Autodesk Inventor part; units mm, degrees
ref_plane "YZ Plane" through (0, 0, 0) normal (1, 0, 0) x (0, 1, 0)
ref_plane "XZ Plane" through (0, 0, 0) normal (0, 1, 0) x (-1, 0, 0)
ref_plane "XY Plane" through (0, 0, 0) normal (0, 0, 1) x (1, 0, 0)
sketch "Skizze1" plane through (0, 0, 0) normal (0, 1, 0) x (-1, 0, 0)
  line L0 (10, -8.25) -> (-10, -8.25)
  line L1 (-10, -8.25) -> (-10, 8.25)
  line L2 (-10, 8.25) -> (10, 8.25)
  line L3 (10, 8.25) -> (10, -8.25)
  line L4 (14, 0) -> (-14, 0)
  line L5 (0, -16.2) -> (0, 37.7)
  circle A0 centre (0, -3.25) radius 3
  line L6 (5, 8.25) -> (-5, 8.25)
  line L7 (-5, 8.25) -> (-5, 16.25)
  line L8 (-5, 16.25) -> (5, 16.25)
  line L9 (5, 16.25) -> (5, 8.25)
  point P0 (0, 0)
  point P1 (-5, 8.25)
  dimension "d0" = 20
  dimension "d1" = 16.5
  dimension "d2" = 6
  dimension "d3" = 11.5
  dimension "d13" = 10
  dimension "d14" = 8
extrude "Extrusion1" add sketch "Skizze1" along normal blind 5 contours L0 L5 A0 L4 L3 | L0 L1 L4 L5 A0 | L4 L5 L2 L3 | L4 L1 L2 L5 | L2 L5 L8 L9 | L2 L7 L8 L5
sketch "Skizze2" plane through (0, 5, 0) normal (0, 1, 0) x (1, 0, 0)
  line L0 (10, -8.25) -> (10, 8.25)
  line L1 (10, 8.25) -> (-10, 8.25)
  line L2 (-10, 8.25) -> (-10, -8.25)
  line L3 (-10, -8.25) -> (-5, -8.25)
  circle A0 centre (0, 3.25) radius 3
  line L4 (-2, -8.25) -> (3, -8.25)
  line L5 (-14, 0) -> (14, 0)
  line L6 (0, 16.2) -> (0, -37.7)
  line L7 (-2.5, -18.25) -> (2.5, -18.25)
  line L8 (2.5, -18.25) -> (2.5, -13.25)
  line L9 (2.5, -13.25) -> (-2.5, -13.25)
  line L10 (-2.5, -13.25) -> (-2.5, -18.25)
  line L11 (-5, -8.25) -> (-5, -16.25)
  line L12 (-5, -16.25) -> (5, -16.25)
  line L13 (5, -16.25) -> (5, -8.25)
  line L14 (5, -8.25) -> (10, -8.25)
  circle A1 centre (0, 3.25) radius 3
  circle A2 centre (0, -21.75) radius 4
  circle A3 centre (0, -21.75) radius 8
  line L15 (0, -13.75) -> (0, 3.25)
  point P0 (0, 0)
  dimension "d10" = 5
  dimension "d11" = 5
  dimension "d12" = 5
  dimension "d21" = 8
  dimension "d22" = 25
  dimension "d23" = 4
extrude "Extrusion2" add sketch "Skizze2" against normal blind 60 contours A3 L6 A2 L7 L8 L12 L13 | L13 L12 L8 A3 | L8 L12 L6 A3 | L8 L7 A2 L6 L12 | A3 L11 L12 L10 L7 A2 L6 | L6 L12 L10 A3 | L6 A2 L7 L10 L12 | A3 L10 L12 L11
properties part number "Absicherung Kugellager"
The model under review builds one solid part; all positions refer to its coordinate system, in mm. A direction names the side the tool comes from. Round coordinates to 2 decimals unless told otherwise and drop trailing zeros. Order: outer loops, then holes, each group sorted by start corner. A loop starts at its lowest first (then second) coordinate and runs counter-clockwise, first axis right, second up. Notation, with made-up numbers: (-37.75, 70) - (-18.75, 70) arc R23 ccw to (-18.75, 83) - close; hole circle Ø3 at (81, 77). An arc over 180 degrees is marked (long way). Use one line per item in the form item = value.
Q1. Clearance check with flat-ended pins moving along their axes: P1, Ø10, axis at x = 6, y = -15.5, coming from the -Z side; P2, Ø4, axis at x = -8.5, y = 2, coming from the +Z side; P3, Ø4, axis at x = 6.5, y = 1.5, coming from the +Z side. State where each tip first meets the part, or that it passes through.
Response values:
P1 = 13.81
P2 = 26.41
P3 = 28.36
Q2. Tool access review of faces 1 (the flat face through (-7, 2, 8.25)), 2 (the cylindrical face through (-1.73, -24.58, 29.56)), 3 (the flat face through (5, 2, 12)): name each direction out of +Z, -Z, +X, -X, +Y, -Y from which nothing blocks a thin tool from reaching the whole face with its end or side.
Response values:
face_1 = -X, +Y, -Y
face_2 = -Y
face_3 = +X, +Y, -Y
Q3. To check wall thickness, follow line 1 (Z direction, x = 0, y = 3.45); line 2 (X direction, y = -35.5, z = 21.75); line 3 (X direction, y = 3.85, z = -3.25). State the ranges of each line that lie inside material, in increasing order.
Response values:
line_1 = -8.25 to -6.25, -0.25 to 17.75, 25.75 to 29.75
line_2 = -8 to -4, 4 to 8
line_3 = -10 to -3, 3 to 10
Q4. Add section A-A on z = 21.75. Give the boundary of the cut face in (x, y), then the cut area to 3 significant figures.
Response values:
outline = (-8, -55) - (-4, -55) - (-4, 5) - (-8, 5) - close; (4, -55) - (8, -55) - (8, 5) - (4, 5) - close
area = 480 mm^2
Q5. Add section C-C on y = -25. Give the boundary of the cut face in (x, z).
Response values:
outline = circle Ø16 at (0, 21.75); hole circle Ø8 at (0, 21.75)
Q6. Add section B-B on x = 0. Give the boundary of the cut face in (y, z), then the cut area to 3 significant figures.
Response values:
outline = (-55, 13.75) - (0, 13.75) - (0, -0.25) - (5, -0.25) - (5, 17.75) - (-55, 17.75) - close; (-55, 25.75) - (5, 25.75) - (5, 29.75) - (-55, 29.75) - close; (0, -8.25) - (5, -8.25) - (5, -6.25) - (0, -6.25) - close
area = 560 mm^2
Q7. Add section D-D on z = -3.25. Give the boundary of the cut face in (x, y), then the cut area to 3 significant figures.
Response values:
outline = (-10, 0) - (-3, 0) - (-3, 5) - (-10, 5) - close; (3, 0) - (10, 0) - (10, 5) - (3, 5) - close
area = 70.0 mm^2
Q8. Mouldability with a two-part tool opening along Z and no side actions: class faces 4 (the flat face through (0, 2, -8.25)), 5 (the flat face through (0, 5, 7)), 6 (the flat face through (8, 2, 8.25)) as pulls with the +Z half, pulls with the -Z half, needs draft (parallel to the pull), parting line crosses it, or undercut.
Response values:
face_4 = pulls with the -Z half
face_5 = needs draft
face_6 = undercut
